from build123d import *

# Parameters (mm, degrees)
F0_R     = 1.85
F0_R_2   = 4
F0_W     = 10.16
F0_H     = 6.35
F0_W_2   = 12.7
F0_W_3   = 6.35
F0_H_2   = 15.24
F0_H_3   = 8.021719
F1_DEPTH = 6.35


with BuildPart() as f1:
    # F0 (on Top) → F1 (new body)
    with BuildSketch(Plane.XY):
        with BuildLine():
            Line((-60.850162, -6.604), (-60.850162, 0))
            Line((-60.850162, 0), (-47.625, 0))
            Line((-47.625, 0), (-47.625, 203.2))
            add(Edge.make_bspline(
                [(-47.625, 203.2), (-31.75, 207.9625), (0, 217.4875), (31.75, 207.9625), (47.625, 203.2)],
                knots=[0, 0, 0, 0, 48.568161, 97.136322, 97.136322, 97.136322, 97.136322], degree=3))
            Line((47.625, 203.2), (47.625, 0))
            Line((47.625, 0), (60.850162, 0))
            Line((60.850162, 0), (60.850162, -6.604))
            Line((60.850162, -6.604), (89.198314, -6.604))
            Line((89.198314, -6.604), (89.198314, 0))
            Line((89.198314, 0), (94.278314, 0))
            Line((94.278314, 0), (94.278314, 38.1))
            Line((94.278314, 38.1), (100.882314, 38.1))
            Line((100.882314, 38.1), (100.882314, 88.9))
            Line((100.882314, 88.9), (94.278314, 88.9))
            Line((94.278314, 88.9), (94.278314, 114.3))
            Line((94.278314, 114.3), (100.882314, 114.3))
            Line((100.882314, 114.3), (100.882314, 165.1))
            Line((100.882314, 165.1), (94.278314, 165.1))
            Line((94.278314, 165.1), (94.278314, 203.2))
            Line((94.278314, 203.2), (58.854451, 279.166719))
            Line((58.854451, 279.166719), (9.525, 279.166719))
            Line((9.525, 279.166719), (9.525, 263.525))
            Line((9.525, 263.525), (20.955, 263.525))
            Line((20.955, 263.525), (20.955, 248.285))
            Line((20.955, 248.285), (9.525, 248.285))
            Line((9.525, 248.285), (9.525, 241.066719))
            Line((9.525, 241.066719), (-9.525, 241.066719))
            Line((-9.525, 241.066719), (-9.525, 279.166719))
            Line((-9.525, 279.166719), (-58.854451, 279.166719))
            Line((-58.854451, 279.166719), (-94.278314, 203.2))
            Line((-94.278314, 203.2), (-94.278314, 165.1))
            Line((-94.278314, 165.1), (-100.882314, 165.1))
            Line((-100.882314, 165.1), (-100.882314, 114.3))
            Line((-100.882314, 114.3), (-94.278314, 114.3))
            Line((-94.278314, 114.3), (-94.278314, 88.9))
            Line((-94.278314, 88.9), (-100.882314, 88.9))
            Line((-100.882314, 88.9), (-100.882314, 38.1))
            Line((-100.882314, 38.1), (-94.278314, 38.1))
            Line((-94.278314, 38.1), (-94.278314, 0))
            Line((-94.278314, 0), (-89.198314, 0))
            Line((-89.198314, 0), (-89.198314, -6.604))
            Line((-89.198314, -6.604), (-60.850162, -6.604))
        make_face()
        with Locations((-80.681092, 9.743146)):
            Circle(F0_R, mode=Mode.SUBTRACT)
        with Locations((-80.681092, 21.056854)):
            Circle(F0_R, mode=Mode.SUBTRACT)
        with Locations((-69.367384, 9.743146)):
            Circle(F0_R, mode=Mode.SUBTRACT)
        with Locations((-75.024238, 15.4)):
            Circle(F0_R_2, mode=Mode.SUBTRACT)
        with Locations((-69.367384, 21.056854)):
            Circle(F0_R, mode=Mode.SUBTRACT)
        with Locations((-75.024238, 63.5)):
            Rectangle(F0_W, F0_H, mode=Mode.SUBTRACT)
        with Locations((69.367384, 9.743146)):
            Circle(F0_R, mode=Mode.SUBTRACT)
        with Locations((75.024238, 15.4)):
            Circle(F0_R_2, mode=Mode.SUBTRACT)
        with Locations((69.367384, 21.056854)):
            Circle(F0_R, mode=Mode.SUBTRACT)
        with Locations((80.681092, 9.743146)):
            Circle(F0_R, mode=Mode.SUBTRACT)
        with Locations((80.681092, 21.056854)):
            Circle(F0_R, mode=Mode.SUBTRACT)
        with Locations((75.024238, 63.5)):
            Rectangle(F0_W, F0_H, mode=Mode.SUBTRACT)
        with Locations((-75.024238, 139.7)):
            Rectangle(F0_W, F0_H, mode=Mode.SUBTRACT)
        with Locations((-74.405786, 200.025)):
            Rectangle(F0_W_2, F0_H, mode=Mode.SUBTRACT)
        with Locations((-17.78, 227.960319)):
            Rectangle(F0_W_3, F0_H_2, mode=Mode.SUBTRACT)
        with Locations((-17.78, 255.905)):
            Rectangle(F0_W_3, F0_H_2, mode=Mode.SUBTRACT)
        with Locations((75.024238, 139.7)):
            Rectangle(F0_W, F0_H, mode=Mode.SUBTRACT)
        with Locations((74.405786, 200.025)):
            Rectangle(F0_W_2, F0_H, mode=Mode.SUBTRACT)
        with Locations((0, 226.895859)):
            Rectangle(F0_W_3, F0_H_3, mode=Mode.SUBTRACT)
        with Locations((17.78, 227.960319)):
            Rectangle(F0_W_3, F0_H_2, mode=Mode.SUBTRACT)
    extrude(amount=F1_DEPTH)


solid = f1.part
The model under review builds one solid part; all positions refer to its coordinate system, in mm. A direction names the side the tool comes from. Round coordinates to 2 decimals unless told otherwise and drop trailing zeros. Loops run counter-clockwise (first coordinate to the right, second up) from the corner with the lowest first, then second, coordinate; pieces in that order, holes last. Notation, with made-up numbers: M 80.25,69.25 L 115.25,69.25 A13 ccw 115.25,74.25 Z; hole C 36.5,54 d9. An arc over 180 degrees is marked long. Answer as a JSON object with one key per item and string values.
Item 1: Clearance check with flat-ended pins moving along their axes: P1, Ø3, axis at x = 69.37, y = 9.74, coming from the +Z side; P2, Ø1.9, axis at y = 106.5, z = 2, coming from the +X side; P3, Ø3, axis at y = -3, z = 2.5, coming from the -X side; P4, Ø3, axis at x = -17, z = 2, coming from the -Y side. State where each tip first meets the part, or that it passes through.
Check sheet entries:
{"P1": "through", "P2": "x = 94.28", "P3": "x = -89.2", "P4": "y = 210.85"}
Item 2: We need section A-A, the plane y = 15.4. State the section outline as (x, z) points (3 decimals).
Check sheet entries:
{"outline": "M -94.278,0 L -79.024,0 L -79.024,6.35 L -94.278,6.35 Z; M -71.024,0 L -47.625,0 L -47.625,6.35 L -71.024,6.35 Z; M 47.625,0 L 71.024,0 L 71.024,6.35 L 47.625,6.35 Z; M 79.024,0 L 94.278,0 L 94.278,6.35 L 79.024,6.35 Z"}
Item 3: We need section C-C, the plane x = -75. State the section outline as (y, z) points (3 decimals), and give its area (3 significant figures).
Check sheet entries:
{"outline": "M -6.604,0 L 11.4,0 L 11.4,6.35 L -6.604,6.35 Z; M 19.4,0 L 60.325,0 L 60.325,6.35 L 19.4,6.35 Z; M 66.675,0 L 136.525,0 L 136.525,6.35 L 66.675,6.35 Z; M 142.875,0 L 196.85,0 L 196.85,6.35 L 142.875,6.35 Z; M 203.2,0 L 244.542,0 L 244.542,6.35 L 203.2,6.35 Z", "area": "1,420 mm2"}
Item 4: We need section B-B, the plane y = 45. State the section outline as (x, z) points (3 decimals).
Check sheet entries:
{"outline": "M -100.882,0 L -47.625,0 L -47.625,6.35 L -100.882,6.35 Z; M 47.625,0 L 100.882,0 L 100.882,6.35 L 47.625,6.35 Z"}
Item 5: We need section D-D, the plane y = 168.5. State the section outline as (x, z) points (3 decimals), and give its area (3 significant figures).
Check sheet entries:
{"outline": "M -94.278,0 L -47.625,0 L -47.625,6.35 L -94.278,6.35 Z; M 47.625,0 L 94.278,0 L 94.278,6.35 L 47.625,6.35 Z", "area": "592 mm2"}
Item 6: Tool access review of faces 5 (the face through (-20.955, 228, 3)), 6 (the face through (-98, 38.1, 3)), 7 (the face through (98, 165.1, 3)), 8 (the face through (66, 138, 0)), 9 (the face through (-9.525, 260, 3)): name each direction out of +Z, -Z, +X, -X, +Y, -Y from which nothing blocks a thin tool from reaching the whole face with its end or side.
Check sheet entries:
{"face 5": "+Z, -Z", "face 6": "+Z, -Z, -X, -Y", "face 7": "+Z, -Z, +X, +Y", "face 8": "-Z, +X, -X, +Y, -Y", "face 9": "+Z, -Z, +Y"}
Item 7: The part is to be moulded in two halves that separate along X. For faces 1 (the face through (98, 88.9, 3)), 2 (the face through (75, 136.525, 3)), 3 (the face through (94.278, 184, 3)), 4 (the face through (-94.278, 184, 3)), say which applies: +X half, -X half, draft (parallel to the pull), parting line (faces both ways), or undercut.
Check sheet entries:
{"face 1": "draft", "face 2": "undercut", "face 3": "+X half", "face 4": "-X half"}
Item 8: For line 1 along X through (y, z) = (199.5, 1.5) (3 decimals); line 2 along X through (y, z) = (138, 0.5) (3 decimals); line 3 along X through (y, z) = (81, 4) (3 decimals), list the stretches that pass through material, from the lowest coordinate up.
Check sheet entries:
{"line 1": "-94.278 to -80.756, -68.056 to -47.625, 47.625 to 68.056, 80.756 to 94.278", "line 2": "-100.882 to -80.104, -69.944 to -47.625, 47.625 to 69.944, 80.104 to 100.882", "line 3": "-100.882 to -47.625, 47.625 to 100.882"}
